```python
from build123d import *

# Parameters (mm, degrees)
SKETCH_W     = 127
SKETCH_H     = 50.8
PAD_DEPTH    = 5.08
SKETCH001_R  = 1.5875
POCKET_DEPTH = 5.081
FILLET_R     = 0.999998
FILLET001_R  = 0.999998
FILLET002_R  = 0.999998


with BuildPart() as part:
    # Sketch → Pad (new body)
    with BuildSketch(Plane.XY):
        Rectangle(SKETCH_W, SKETCH_H)
    extrude(amount=PAD_DEPTH)

    # Sketch001 (on Face6 of Pad) → Pocket (cut, through all)
    with BuildSketch(Plane.XY.offset(5.08)):
        with Locations((57.15, 12.7)):
            Circle(SKETCH001_R)
        with Locations((57.15, -15.567334)):
            Circle(SKETCH001_R)
        Polygon((-54.077858, -21.3868), (47.585089, -21.3868), (47.585089, 19.226009), align=None)
        Polygon((42.176147, 21.3868), (-59.4868, 21.3868), (-59.4868, -19.226009), align=None)
    extrude(amount=-POCKET_DEPTH, mode=Mode.SUBTRACT)

    # Fillet
    fillet_edges = [part.edges().sort_by_distance(p)[0] for p in [
        (-59.4868, 21.3868, 2.54),
        (47.585089, -21.3868, 2.54),
    ]]
    fillet(fillet_edges, radius=FILLET_R)

    # Fillet001
    fillet001_edges = [part.edges().sort_by_distance(p)[0] for p in [
        (-54.077858, -21.3868, 2.54),
        (42.176147, 21.3868, 2.54),
    ]]
    fillet(fillet001_edges, radius=FILLET001_R)

    # Fillet002
    fillet002_edges = [part.edges().sort_by_distance(p)[0] for p in [
        (47.585089, 19.226009, 2.54),
        (-59.4868, -19.226009, 2.54),
    ]]
    fillet(fillet002_edges, radius=FILLET002_R)


solid = part.part
```
Geometry check sheet. Reference: the model listing, model coordinates, mm. A direction names the side the tool comes from. Give positions to 0.01 mm unless a question says otherwise; leave off trailing zeros. Loops run counter-clockwise (first coordinate to the right, second up) from the corner with the lowest first, then second, coordinate; pieces in that order, holes last. Notation, with made-up numbers: (63.25, 36) - (75.25, 36) arc R20 ccw to (75.25, 49) - close; hole circle Ø7 at (25.5, 52). An arc over 180 degrees is marked (long way). Use CSV: the item, a comma, the result in double quotes. Start each with the question number.
Q1. Section check B-B, the plane y = 12.7. Record the cut outline in (x, z), and give its area (3 significant figures).
Q2. Section check A-A, the plane x = 57.15. Record the cut outline in (y, z), and give its area (3 significant figures).
Q3. Scan lines: probe 1 along Y at (x, z) = (57.15, 2.4); probe 2 along Y at (x, z) = (8.5, 4.8); probe 3 along Y at (x, z) = (46, 0.6). Record each from-to range of solid material in increasing order. Write a range as from..to.
Q4. Release check for a two-part mould opening along Y. For faces 3 (the face through (63.5, 0, 3)), 4 (the face through (-59.487, 2, 3)), 5 (the face through (-1, 25.4, 3)) record: +Y half, -Y half, draft (parallel to the pull), parting line (faces both ways), or undercut.
Q5. Section check C-C, the plane z = 2.35. Count the separate pieces of the cut face and the enclosed holes in it, and give its area (3 significant figures).
Q6. Access from +Z, -Z, +X, -X, +Y, -Y to the whole of each face (thin tool, end or side, straight path). Record for faces 1 (the face through (-0.85, -0.123, 2.576)), 2 (the face through (-63.5, 0, 3)).
Q7. Section check D-D, the plane x = 0.5. Record the cut outline in (y, z), and give its area (3 significant figures).
Findings below:
1,outline,"(-63.5, 0) - (-59.49, 0) - (-59.49, 5.08) - (-63.5, 5.08) - close; (20.43, 0) - (31.25, 0) - (31.25, 5.08) - (20.43, 5.08) - close; (47.59, 0) - (55.56, 0) - (55.56, 5.08) - (47.59, 5.08) - close; (58.74, 0) - (63.5, 0) - (63.5, 5.08) - (58.74, 5.08) - close"
1,area,"140 mm^2"
2,outline,"(-25.4, 0) - (-17.15, 0) - (-17.15, 5.08) - (-25.4, 5.08) - close; (-13.98, 0) - (11.11, 0) - (11.11, 5.08) - (-13.98, 5.08) - close; (14.29, 0) - (25.4, 0) - (25.4, 5.08) - (14.29, 5.08) - close"
2,area,"226 mm^2"
3,probe 1,"y = -25.4..-17.15, -13.98..11.11, 14.29..25.4"
3,probe 2,"y = -25.4..-21.39, 3.61..7.93, 21.39..25.4"
3,probe 3,"y = -25.4..-21.39, 18.59..25.4"
4,face 3,"draft"
4,face 4,"undercut"
4,face 5,"+Y half"
5,separate pieces,"1"
5,enclosed holes,"4"
5,area,"2,320 mm^2"
6,face 1,"+Z, -Z"
6,face 2,"+Z, -Z, -X, +Y, -Y"
7,outline,"(-25.4, 0) - (-21.39, 0) - (-21.39, 5.08) - (-25.4, 5.08) - close; (0.42, 0) - (4.74, 0) - (4.74, 5.08) - (0.42, 5.08) - close; (21.39, 0) - (25.4, 0) - (25.4, 5.08) - (21.39, 5.08) - close"
7,area,"62.7 mm^2"
